```python
from build123d import *

# Parameters (mm, degrees)
SKETCH1_R               = 21.082
SKETCH1_R_2             = 17.272
BOSS_EXTRUDE1_DEPTH     = 1160.4625
F_1_4_CLEARANCE_HOLE1_D = 6.7564


with BuildPart() as part:
    # Sketch1 → Boss-Extrude1 (new body)
    with BuildSketch(Plane(origin=(0, 0, 0), x_dir=(1, 0, 0), z_dir=(0, 1, 0))):
        Circle(SKETCH1_R)
        Circle(SKETCH1_R_2, mode=Mode.SUBTRACT)
    extrude(amount=BOSS_EXTRUDE1_DEPTH)

    # 1/4 Clearance Hole1 (through all)
    with Locations(Plane.XY.offset(21.082)):
        with Locations((0, 15.875), (0, 66.675)):
            Hole(F_1_4_CLEARANCE_HOLE1_D / 2)


solid = part.part
```
Design review of the part built by this model. Coordinates are the model's own, in mm. Coordinates: 2 decimals unless noted, no trailing zeros. Loops run counter-clockwise (first coordinate to the right, second up) from the corner with the lowest first, then second, coordinate; pieces in that order, holes last.
Q1. The part is to be moulded in two halves that separate along X. For faces 1 (the face through (-8, 1160.462, 16)), 2 (the face through (20.11, 572.11, -6.33)), 3 (the face through (-2.248, 572.108, -17.125)), say which applies: +X half, -X half, draft (parallel to the pull), parting line (faces both ways), or undercut.
Reported:
face 1: draft
face 2: parting line
face 3: undercut
Q2. We need section B-B on y = 245. State the section outline as (x, z) points, and give its area (3 significant figures).
Reported:
outline: circle Ø42.16 at (0, 0); hole circle Ø34.54 at (0, 0)
area: 459 mm2
Q3. For pin 1 (10 mm diameter, centred on x = 0, z = -7.5, fed in from -Y); pin 2 (8 mm diameter, centred on x = 10.5, z = 12, fed in from +Y); pin 3 (8 mm diameter, centred on y = 791.5, z = 7.5, fed in from +X); pin 4 (1.5 mm diameter, centred on y = 520.5, z = -16.5, fed in from +X), all flat-tipped, find the tip position at first contact; note any pin that passes through.
Reported:
pin 1: passes through
pin 2: stops at y = 1160.46
pin 3: stops at x = 20.79
pin 4: stops at x = 14.01
Q4. We need section A-A on z = 0. State the section outline as (x, y) points, and give its area (3 significant figures).
Reported:
outline: (-21.08, 0) - (-17.27, 0) - (-17.27, 1160.46) - (-21.08, 1160.46) - close; (17.27, 0) - (21.08, 0) - (21.08, 1160.46) - (17.27, 1160.46) - close
area: 8,840 mm2
Q5. To check wall thickness, follow line 1 (Y direction, x = 0, z = 19); line 2 (Z direction, x = -1.5, y = 528.5); line 3 (X direction, y = 927, z = 0). State the ranges of each line that lie inside material, in increasing order.
Reported:
line 1: y = 0 to 12.5, 19.25 to 63.3, 70.05 to 1160.46
line 2: z = -21.03 to -17.21, 17.21 to 21.03
line 3: x = -21.08 to -17.27, 17.27 to 21.08
